Source: three-view drawing plus pictorial views. Frame: mm from the lowest corner of the part. A direction names the side the tool comes from. Give positions to 0.01 mm unless a question says otherwise; leave off trailing zeros. Order: outer loops, then holes, each group sorted by start corner. A loop starts at its lowest first (then second) coordinate and runs counter-clockwise, first axis right, second up. Notation, with made-up numbers: M 0,-40 L 49,-40 A19 ccw 49,-33 Z; hole C 48.25,47 d5. An arc over 180 degrees is marked long. Use CSV: the item, a comma, the result in double quotes. Start each with the question number.
1. Reachability of the marked faces 4 and 5 from +Z, -Z, +X, -X, +Y, -Y: full face, straight path, thin tool, end or side. Return the list, or none.
2. Section query B-B, the plane x = 17.5. Return the cut outline in (y, z), plus the area to 3 significant figures.
3. Pin query (flat end, axial travel): P1, Ø2.5, axis at x = 31.5, z = 11, coming from the -Y side; P2, Ø8, axis at x = 20.5, y = 15.5, coming from the -Z side; P3, Ø4, axis at x = 21.5, y = 2.5, coming from the +Z side; P4, Ø7, axis at y = 18.5, z = 9, coming from the -X side. Return the tip coordinate at first contact, or that it passes through.
4. Section query D-D, the plane y = 3.75. Return the cut outline in (x, z).
5. Mould query, pull axis Z, two halves, no side actions, for the marked faces 1, 2 and 3. Classes: released by +Z, released by -Z, zero draft, split by the parting line, or undercut.
6. Line query: line 1 along Y through (x, z) = (17.5, 2.75); line 2 along X through (y, z) = (4, 12.5); line 3 along Z through (x, y) = (13, 9.75). Output: solid intervals per line, ascending. Write a range as [from, to].
7. Section query C-C, the plane z = 1.5. Return the cut outline in (x, y), plus the area to 3 significant figures.
8. Section query A-A, the plane y = 12.5. Return the cut outline in (x, z), plus the area to 3 significant figures.
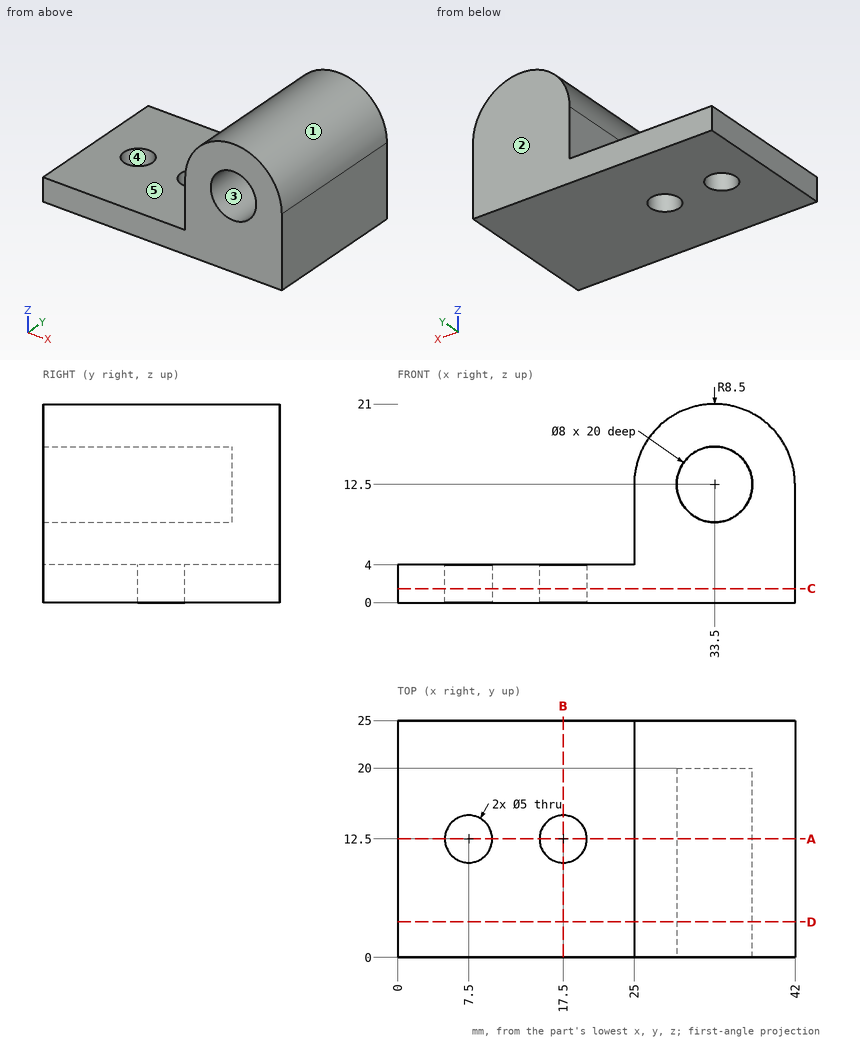
Result set:
1,face 4,"+Z, -Z"
1,face 5,"+Z, -X, +Y, -Y"
2,outline,"M 0,0 L 10,0 L 10,4 L 0,4 Z; M 15,0 L 25,0 L 25,4 L 15,4 Z"
2,area,"80.0 mm2"
3,P1,"y = 20"
3,P2,"z = 0"
3,P3,"z = 4"
3,P4,"x = 25"
4,outline,"M 0,0 L 42,0 L 42,12.5 A8.5 ccw 25,12.5 L 25,4 L 0,4 Z; hole C 33.5,12.5 d8"
5,face 1,"released by +Z"
5,face 2,"zero draft"
5,face 3,"undercut"
6,line 1,"[0, 10], [15, 25]"
6,line 2,"[25, 29.5], [37.5, 42]"
6,line 3,"[0, 4]"
7,outline,"M 0,0 L 42,0 L 42,25 L 0,25 Z; hole C 7.5,12.5 d5; hole C 17.5,12.5 d5"
7,area,"1,010 mm2"
8,outline,"M 0,0 L 5,0 L 5,4 L 0,4 Z; M 10,0 L 15,0 L 15,4 L 10,4 Z; M 20,0 L 42,0 L 42,12.5 A8.5 ccw 25,12.5 L 25,4 L 20,4 Z; hole C 33.5,12.5 d8"
8,area,"336 mm2"
